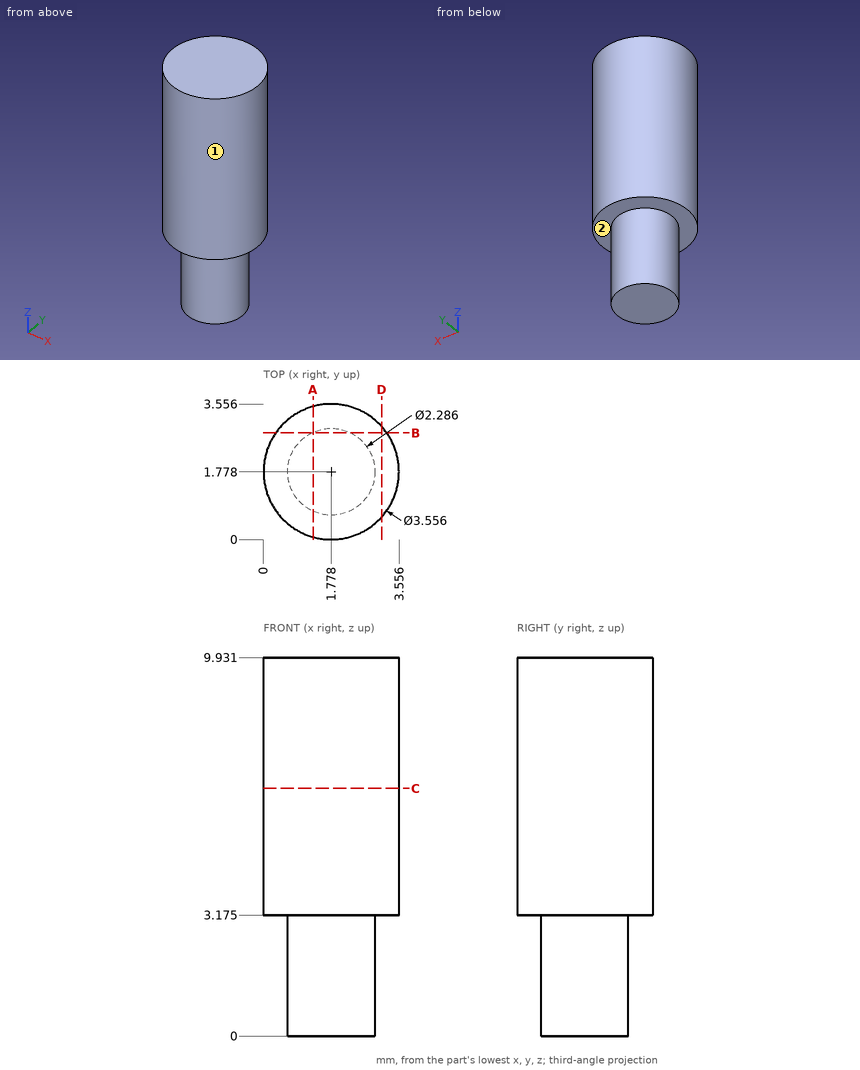
For this review, use the dimensioned drawing (mm, ordinates from the lowest corner) and the shaded views. A direction names the side the tool comes from. Coordinates: 2 decimals unless noted, no trailing zeros. Loops run counter-clockwise (first coordinate to the right, second up) from the corner with the lowest first, then second, coordinate; pieces in that order, holes last. Notation, with made-up numbers: (20, 73.25) -> (77, 73.25) arc R12 ccw to (77, 89.25) -> close; hole circle Ø2 at (51, 19). An arc over 180 degrees is marked (long way). Use a Markdown table: item, result. Add a question column.
Item 1: Wall thickness on L1, parallel to Z at x = 3.35, y = 2.4 (1 decimal); L2, parallel to Y at x = 1.7, z = 6 (1 decimal); L3, parallel to Y at x = 2.4, z = 2.5: over which ranges is each line inside the solid? List them lowest first. Write a range as from..to.
Item 2: Clearance check with a flat-ended pin moving along its axis: P1, Ø2, axis at x = 2.5, z = 1.5, coming from the +Y side. State where the tip first meets the part, or that it passes through.
Item 3: We need section A-A, the plane x = 1.3. Write out the cut boundary in (y, z) (1 decimal).
Item 4: We need section D-D, the plane x = 3.1. Write out the cut boundary in (y, z) (1 decimal).
Item 5: We need section B-B, the plane y = 2.8. Write out the cut boundary in (x, z) (1 decimal).
Item 6: We need section C-C, the plane z = 6.5. Write out the cut boundary in (x, y).
Item 7: Machinability: for the marked faces 1 and 2, which of the approach directions +Z, -Z, +X, -X, +Y, -Y give a long, thin tool a straight path to every point of the face, cutting with its end or side? Answer none if there is none.
Numbers:
| question | item | result |
|---|---|---|
| 1 | L1 | z = 3.2..9.9 |
| 1 | L2 | y = 0..3.6 |
| 1 | L3 | y = 0.82..2.74 |
| 2 | P1 | stops at y = 2.92 |
| 3 | outline | (0.1, 3.2) -> (0.7, 3.2) -> (0.7, 0) -> (2.8, 0) -> (2.8, 3.2) -> (3.5, 3.2) -> (3.5, 9.9) -> (0.1, 9.9) -> close |
| 4 | outline | (0.6, 3.2) -> (3, 3.2) -> (3, 9.9) -> (0.6, 9.9) -> close |
| 5 | outline | (0.3, 3.2) -> (1.3, 3.2) -> (1.3, 0) -> (2.3, 0) -> (2.3, 3.2) -> (3.2, 3.2) -> (3.2, 9.9) -> (0.3, 9.9) -> close |
| 6 | outline | circle Ø3.56 at (1.78, 1.78) |
| 7 | face 1 | +Z, -Z |
| 7 | face 2 | -Z |
